The listing builds one solid part. Answer for the finished solid, in the listing's coordinates (mm). A direction names the side the tool comes from. Give positions to 0.01 mm unless a question says otherwise; leave off trailing zeros. Order: outer loops, then holes, each group sorted by start corner. A loop starts at its lowest first (then second) coordinate and runs counter-clockwise, first axis right, second up. Notation, with made-up numbers: (13.5, 80.25) - (52.5, 80.25) arc R8 ccw to (52.5, 93.25) - close; hole circle Ø7 at (47, 58). An arc over 180 degrees is marked (long way). Answer as a JSON object with one key per item and string values. Group by question number.
Q1. A cutting plane is placed at B-B, the plane z = 96.5. Give the vertices of the cut face in (x, y) (1 decimal).
Q2. For faces 1 (the face through (-0.02, -20.95, 22.51)), 2 (the face through (-1.588, -19, 48)), 3 (the face through (0.022, -33.855, -37.109)), determine the directions among +Z, -Z, +X, -X, +Y, -Y from which every point of the face is accessible in a straight line to the end or side of a thin tool.
Q3. Consider line 1 (Y direction, x = -0.05, z = 80) (3 decimals); line 2 (Z direction, x = -1, y = 12) (3 decimals); line 3 (Z direction, x = 0.9, y = 7). Determine where each line is inside the solid, lowest interval first.
Q4. The mould has two halves that part along Z. Classify faces 4 (the face through (-0.022, 6.776, 69.574)), 5 (the face through (0, -66, 94.7)), 6 (the face through (-0.022, -15.141, 132.384)): released by +Z, released by -Z, zero draft, split by the parting line, or undercut.
Q5. Given pin 1 (1.5 mm diameter, centred on x = -1, z = -9.5, fed in from +Y); pin 2 (1 mm diameter, centred on x = -0.5, z = -64, fed in from +Y), each flat-ended and moving along its own axis, determine where each tip first touches the part or whether it passes through.
Q6. A cutting plane is placed at C-C, the plane y = -55. Give the vertices of the cut face in (x, z).
Q7. A cutting plane is placed at A-A, the plane y = -7.5. Give the vertices of the cut face in (x, z), and give its area (3 significant figures).
Q8. A cutting plane is placed at D-D, the plane x = -0.45. Count the separate pieces of the cut face and the enclosed holes in it, and give its area (3 significant figures).
from build123d import *

# Parameters (mm, degrees)
SKETCH1_R                  = 4.7625
SKETCH1_R_2                = 11.1125
BOSS_EXTRUDE1_DEPTH        = 1.5875
SKETCH12_R                 = 11.1125
BOSS_EXTRUDE2_DEPTH        = 1.5875
F_6_CLEARANCE_HOLE1_D      = 3.6576
M3X0_5_TAPPED_HOLE1_D      = 2.5
M4_CLEARANCE_HOLE1_D       = 4.5
M2X0_4_TAPPED_HOLE1_D      = 1.6
FILLET1_R                  = 5
FILLET2_R                  = 3.175
CUT_EXTRUDE1_DEPTH         = 155.713872435
CUT_EXTRUDE1_DEPTH_BACK    = 155.713872435
SKETCH1_3_R                = 2
F_1_4_0_2500_DOWEL_HOLE1_D = 6.35
F_1_5MM_START              = -1.5875
F_1_5MM_DOWEL_SLOT1_DEPTH  = 3.175
M2_5X0_45_TAPPED_HOLE1_D   = 2.05


# Read off the part's stored shape, not the designer's step: Ø1.5mm Dowel Slot1
with BuildPart() as part:
    # Sketch1 → Boss-Extrude1 (new, symmetric)
    with BuildSketch(Plane(origin=(0, 0, 0), x_dir=(0, 0, -1), z_dir=(1, 0, 0))):
        with BuildLine():
            ThreePointArc((-83.281063832, -19.348369622), (-96.105900293, -64.061735294), (-49.900079745, -69.426774672))
            Line((-49.900079745, -69.426774672), (11.366191703, -12.160004571))
            ThreePointArc((11.366191703, -12.160004571), (15.483205435, 6.109531443), (0, 16.645))
            Line((0, 16.645), (-133.81, 16.645))
            Line((-133.81, 16.645), (-133.81, -16.645))
            Line((-133.81, -16.645), (-77.295250897, -16.645))
            Line((-77.295250897, -16.645), (-83.281063832, -19.348369622))
        make_face()
        with Locations((-70.72728593, -47.145)):
            Circle(SKETCH1_R, mode=Mode.SUBTRACT)
        Circle(SKETCH1_R_2, mode=Mode.SUBTRACT)
    extrude(amount=BOSS_EXTRUDE1_DEPTH, both=True)

    # Sketch12 → Boss-Extrude2 (add, symmetric)
    with BuildSketch(Plane(origin=(0, 0, 0), x_dir=(0, 0, -1), z_dir=(1, 0, 0))):
        with BuildLine():
            Line((83.375435824, -22.327935442), (6.339273926, 13.594616806))
            ThreePointArc((6.339273926, 13.594616806), (-13.594616806, 6.339273926), (-6.339273926, -13.594616806))
            Line((-6.339273926, -13.594616806), (70.696887972, -49.517169054))
            ThreePointArc((70.696887972, -49.517169054), (90.630778704, -42.261826174), (83.375435824, -22.327935442))
        make_face()
        Circle(SKETCH12_R, mode=Mode.SUBTRACT)
    extrude(amount=BOSS_EXTRUDE2_DEPTH, both=True)

    # #6 Clearance Hole1 (through all)
    with Locations(Plane(origin=(1.5875, 0, 0), x_dir=(0, 0, -1), z_dir=(1, 0, 0))):
        with Locations((-80, -13.475), (-80, 13.475), (-130, 13.475), (-130, -13.475)):
            Hole(F_6_CLEARANCE_HOLE1_D / 2)

    # M3x0.5 Tapped Hole1 (through all)
    with Locations(Plane(origin=(1.5875, 0, 0), x_dir=(0, 0, -1), z_dir=(1, 0, 0))):
        with Locations((-53.003557214, -40.529688942), (-69.983650742, -28.241563627)):
            Hole(M3X0_5_TAPPED_HOLE1_D / 2)

    # M4 Clearance Hole1 (through all)
    with Locations(Plane(origin=(1.5875, 0, 0), x_dir=(0, 0, -1), z_dir=(1, 0, 0))):
        with Locations((84.362778856, -42.728482305), (-69.34493086, -68.600514314), (-89.999483912, -37.614397451), (67.478745093, -38.864623629)):
            Hole(M4_CLEARANCE_HOLE1_D / 2)

    # M2x0.4 Tapped Hole1 (through all)
    with Locations(Plane(origin=(1.5875, 0, 0), x_dir=(0, 0, -1), z_dir=(1, 0, 0))):
        with Locations((-33.212044815, -37.265281486), (-40.152269713, -43.752444068)):
            Hole(M2X0_4_TAPPED_HOLE1_D / 2)

    # Fillet1
    fillet1_edges = [part.edges().sort_by_distance(p)[0] for p in [
        (0, -16.645, 133.81),
        (0, 16.645, 133.81),
    ]]
    fillet(fillet1_edges, radius=FILLET1_R)

    # Fillet2
    fillet2_edges = [part.edges().sort_by_distance(p)[0] for p in [
        (0, -16.645, 77.295250897),
    ]]
    fillet(fillet2_edges, radius=FILLET2_R)

    # Sketch1<3> → Cut-Extrude1 (cut, two sides: drawn at the far end of the back side and taken through both)
    with BuildSketch(Plane(origin=(0, 0, 0), x_dir=(0, 0, -1), z_dir=(1, 0, 0)).offset(-CUT_EXTRUDE1_DEPTH_BACK)):
        with Locations((-80, -19.435)):
            Circle(SKETCH1_3_R)
    extrude(amount=CUT_EXTRUDE1_DEPTH + CUT_EXTRUDE1_DEPTH_BACK, mode=Mode.SUBTRACT)

    # 1/4 (0.2500) Dowel Hole1 (through all)
    with Locations(Plane(origin=(1.5875, 0, 0), x_dir=(0, 0, -1), z_dir=(1, 0, 0))):
        with Locations((-66.545805833, 5.822003616)):
            Hole(F_1_4_0_2500_DOWEL_HOLE1_D / 2)

    # Ø1.5mm Dowel Slot1 outline → Ø1.5mm Dowel Slot1 (cut)
    with BuildSketch(Plane.YZ.offset(F_1_5MM_START)):
        with BuildLine():
            Line((-16.249877423, 11.160935612), (-10.040202515, 16.965238975))
            ThreePointArc((-10.040202515, 16.965238975), (-10.004434437, 18.025295881), (-11.064491343, 18.061063959))
            Line((-11.064491343, 18.061063959), (-17.274166252, 12.256760596))
            ThreePointArc((-17.274166252, 12.256760596), (-17.30993433, 11.196703689), (-16.249877423, 11.160935612))
        make_face()
        with BuildLine():
            Line((-23.078469615, 18.466435504), (-16.868794706, 24.270738867))
            ThreePointArc((-16.868794706, 24.270738867), (-16.833026629, 25.330795773), (-17.893083535, 25.366563851))
            Line((-17.893083535, 25.366563851), (-24.102758444, 19.562260488))
            ThreePointArc((-24.102758444, 19.562260488), (-24.138526521, 18.502203582), (-23.078469615, 18.466435504))
        make_face()
    extrude(amount=F_1_5MM_DOWEL_SLOT1_DEPTH, mode=Mode.SUBTRACT)

    # M2.5x0.45 Tapped Hole1 (through all)
    with Locations(Plane(origin=(1.5875, 0, 0), x_dir=(0, 0, -1), z_dir=(1, 0, 0))):
        with Locations((-35, 2.5), (-25, 2.5)):
            Hole(M2_5X0_45_TAPPED_HOLE1_D / 2)


solid = part.part
Reply:
{
 "1": {"outline": "(-1.6, -63.5) - (1.6, -63.5) - (1.6, -30.8) - (-1.6, -30.8) - close; (-1.6, -16.6) - (1.6, -16.6) - (1.6, 16.6) - (-1.6, 16.6) - close"},
 "2": {"face 1": "+X, -X", "face 2": "+Z, -Z, -X, +Y, -Y", "face 3": "+X, -X, -Y"},
 "3": {"line 1": "y = -76.201 to -21.435, -17.435 to -15.304, -11.646 to 11.646, 15.304 to 16.645", "line 2": "z = -11.535 to 78.919, 81.081 to 128.919, 131.081 to 133.797", "line 3": "z = -20.48 to -8.63, 8.63 to 63.6, 69.49 to 133.81"},
 "4": {"face 4": "undercut", "face 5": "split by the parting line", "face 6": "released by +Z"},
 "5": {"pin 1": "stops at y = 14.16", "pin 2": "stops at y = -13.06"},
 "6": {"outline": "(-1.59, 34.47) - (1.59, 34.47) - (1.59, 100.2) - (-1.59, 100.2) - close"},
 "7": {"outline": "(-1.59, -51.58) - (1.59, -51.58) - (1.59, -8.2) - (-1.59, -8.2) - close; (-1.59, 8.2) - (1.59, 8.2) - (1.59, 133.81) - (-1.59, 133.81) - close", "area": "537 mm^2"},
 "8": {"separate pieces": "1", "enclosed holes": "20", "area": "10,900 mm^2"}
}
